from build123d import *

# Parameters (mm, degrees)
BOX033_W              = 10
BOX033_H              = 10
BOX033_DEPTH          = 18
CYLINDER011_R         = 3.15
CYLINDER011_DEPTH     = 10
CYLINDER012_R         = 6
CYLINDER012_DEPTH     = 10
BOX026_W              = 6
BOX026_H              = 16
BOX026_DEPTH          = 16
BOX027_W              = 1
BOX027_H              = 7.8
BOX027_DEPTH          = 16
CHAMFER006006011_SIZE = 0.99
CHAMFER006006012_SIZE = 2
CHAMFER006006013_SIZE = 0.4


with BuildPart() as cube032:
    # Box033 → Box033 (new body)
    with BuildSketch(Plane(origin=(-3.5, 22, -12.5), x_dir=(1, 0, 0), z_dir=(0, 0, 1))):
        with Locations((5, 5)):
            Rectangle(BOX033_W, BOX033_H)
    extrude(amount=BOX033_DEPTH)


with BuildPart() as cylinder011:
    # Cylinder011 → Cylinder011 (new body)
    with BuildSketch(Plane(origin=(2, 15, 8), x_dir=(0, 0, 1), z_dir=(-1, 0, 0))):
        Circle(CYLINDER011_R)
    extrude(amount=CYLINDER011_DEPTH)


with BuildPart() as fusion005:
    # Cylinder012 → Cylinder012 (new body)
    with BuildSketch(Plane(origin=(-5, 15, 8), x_dir=(0, 0, 1), z_dir=(-1, 0, 0))):
        Circle(CYLINDER012_R)
    extrude(amount=CYLINDER012_DEPTH)

    # Fusion005: union Cylinder011
    add(cylinder011.part)


with BuildPart() as cube025:
    # Box026 → Box026 (new body)
    with BuildSketch(Plane(origin=(-6, 7, 0), x_dir=(1, 0, 0), z_dir=(0, 0, 1))):
        with Locations((3, 8)):
            Rectangle(BOX026_W, BOX026_H)
    extrude(amount=BOX026_DEPTH)


with BuildPart() as cut002004005004:
    # Box027 → Box027 (new body)
    with BuildSketch(Plane(origin=(0, 11.1, 0), x_dir=(1, 0, 0), z_dir=(0, 0, 1))):
        with Locations((0.5, 3.9)):
            Rectangle(BOX027_W, BOX027_H)
    extrude(amount=BOX027_DEPTH)

    # Fusion006: union Cube025
    add(cube025.part)

    # Cut002004002: cut Fusion005
    add(fusion005.part, mode=Mode.SUBTRACT)

    # Chamfer006006011
    chamfer006006011_edges = [cut002004005004.edges().sort_by_distance(p)[0] for p in [
        (-6, 15, 2),
    ]]
    chamfer(chamfer006006011_edges, length=CHAMFER006006011_SIZE)

    # Chamfer006006012
    chamfer006006012_edges = [cut002004005004.edges().sort_by_distance(p)[0] for p in [
        (-3, 7, 0),
        (-3, 7, 16),
        (-3, 23, 16),
        (-3, 23, 0),
    ]]
    chamfer(chamfer006006012_edges, length=CHAMFER006006012_SIZE)

    # Chamfer006006013
    chamfer006006013_edges = [cut002004005004.edges().sort_by_distance(p)[0] for p in [
        (-6, 7, 8),
        (-6, 8, 1),
        (-6, 15, 0),
        (-6, 22, 1),
        (-6, 23, 8),
        (-6, 22, 15),
        (-6, 15, 16),
        (-6, 8, 15),
    ]]
    chamfer(chamfer006006013_edges, length=CHAMFER006006013_SIZE)


with BuildPart() as cut002004005004_1:
    # Chamfer006006013 placement: moved
    add(cut002004005004.part.moved(Location((0, 0, -11))))

    # Cut002004005004: cut Cube032
    add(cube032.part, mode=Mode.SUBTRACT)


solid = cut002004005004_1.part
Geometry: final body of the model. Coordinates: model frame, mm. A direction names the side the tool comes from. Coordinates: 2 decimals unless noted, no trailing zeros. Order: outer loops, then holes, each group sorted by start corner. A loop starts at its lowest first (then second) coordinate and runs counter-clockwise, first axis right, second up.
1) Draft query along Z for faces 4 (the flat face through (-2, 15, 5)), 5 (the cylindrical face through (-1.958, 11.925, -3.683)), 6 (the flat face through (-5.8, 8.13, -9.85)). Return one class per face: released by +Z, released by -Z, zero draft, split by the parting line, or undercut.
Result sheet:
face 4: released by +Z
face 5: undercut
face 6: released by -Z
2) First-contact query: P1, Ø0.8, axis at x = 0.5, z = -3, coming from the +Y side; P2, Ø8, axis at y = 15, z = -3, coming from the -X side; P3, Ø4.5, axis at y = 8.5, z = -6.5, coming from the +X side. Flat tips, straight axial feed; report the tip coordinate or a pass-through.
Result sheet:
P1: stops at y = 18.9
P2: stops at x = -5
P3: stops at x = 0
3) Set-up query: faces 1 (the flat face through (-3, 7, -3)), 2 (the flat face through (0, 9, -3)), 3 (the flat face through (-3.5, 22.5, -3.1)). Return all of +Z, -Z, +X, -X, +Y, -Y with unobstructed straight access to the full face (end or side cutting, diameter ignored); none if empty.
Result sheet:
face 1: +Z, -Z, +X, -X, -Y
face 2: +Z, -Z, +X, -Y
face 3: +Z, -Z, +X, +Y
4) Section C-C (x = -4.5). Return loops of the section in (y, z).
Result sheet:
outline: (7, -9) - (9, -11) - (21, -11) - (23, -9) - (23, 3) - (21, 5) - (9, 5) - (7, 3) - close; hole circle Ø6.3 at (15, -3)
5) Section D-D (x = -2.5). Return loops of the section in (y, z), then the cut area to 3 significant figures.
Result sheet:
outline: (7, -9) - (9, -11) - (21, -11) - (22, -10) - (22, 4) - (21, 5) - (9, 5) - (7, 3) - close; hole circle Ø6.3 at (15, -3)
area: 204 mm2
6) Ray query, probe 1 along Y at (x, z) = (-2.2, -3); probe 2 along Z at (x, y) = (-4.95, 15); probe 3 along Y at (x, z) = (-4.95, -3). Return the intervals inside material, ascending.
Result sheet:
probe 1: y = 7 to 11.85, 18.15 to 22
probe 2: z = -11 to -6.15, 0.15 to 5
probe 3: y = 7 to 11.85, 18.15 to 23
